Build history of the part. All positions in model axes, mm. Give positions to 0.01 mm unless a question says otherwise; leave off trailing zeros. Loops run counter-clockwise (first coordinate to the right, second up) from the corner with the lowest first, then second, coordinate; pieces in that order, holes last. Notation, with made-up numbers: (-30.75, -21.75) -> (13.25, -21.75) arc R10 cw to (13.25, -12.75) -> close; hole circle Ø5 at (51.25, -10.75). An arc over 180 degrees is marked (long way). Answer in a Markdown table with one row per item. Add a question column.
from build123d import *

# Parameters (mm, degrees)
SKETCH1_W           = 180
SKETCH1_H           = 9.9
BOSS_EXTRUDE1_DEPTH = 4.9
SKETCH2_R           = 1.65
CUT_EXTRUDE1_DEPTH  = 5.9
CUT_EXTRUDE2_DEPTH  = 2.2


with BuildPart() as part:
    # Sketch1 → Boss-Extrude1 (new body)
    with BuildSketch(Plane.XY):
        with Locations((-56.357347179, 33.440788785)):
            Rectangle(SKETCH1_W, SKETCH1_H)
    extrude(amount=-BOSS_EXTRUDE1_DEPTH)

    # Sketch2 → Cut-Extrude1 (cut, through all)
    with BuildSketch(Plane.XY):
        with Locations((-136.357347179, 33.440788785)):
            Circle(SKETCH2_R)
        with Locations((-66.357347179, 33.440788785)):
            Circle(SKETCH2_R)
        with Locations((-46.357347179, 33.440788785)):
            Circle(SKETCH2_R)
        with Locations((23.642652821, 33.440788785)):
            Circle(SKETCH2_R)
    extrude(amount=-CUT_EXTRUDE1_DEPTH, mode=Mode.SUBTRACT)

    # Sketch3 → Cut-Extrude2 (cut)
    with BuildSketch(Plane.XY):
        Polygon((-134.711898912, 30.590788785), (-133.066450645, 33.440788785), (-134.711898912, 36.290788785), (-138.002795446, 36.290788785), (-139.648243713, 33.440788785), (-138.002795446, 30.590788785), align=None)
        Polygon((-64.711898912, 30.590788785), (-63.066450645, 33.440788785), (-64.711898912, 36.290788785), (-68.002795446, 36.290788785), (-69.648243713, 33.440788785), (-68.002795446, 30.590788785), align=None)
        Polygon((-44.711898912, 30.590788785), (-43.066450645, 33.440788785), (-44.711898912, 36.290788785), (-48.002795446, 36.290788785), (-49.648243713, 33.440788785), (-48.002795446, 30.590788785), align=None)
        Polygon((25.288101088, 30.590788785), (26.933549355, 33.440788785), (25.288101088, 36.290788785), (21.997204554, 36.290788785), (20.351756287, 33.440788785), (21.997204554, 30.590788785), align=None)
    extrude(amount=-CUT_EXTRUDE2_DEPTH, mode=Mode.SUBTRACT)


solid = part.part
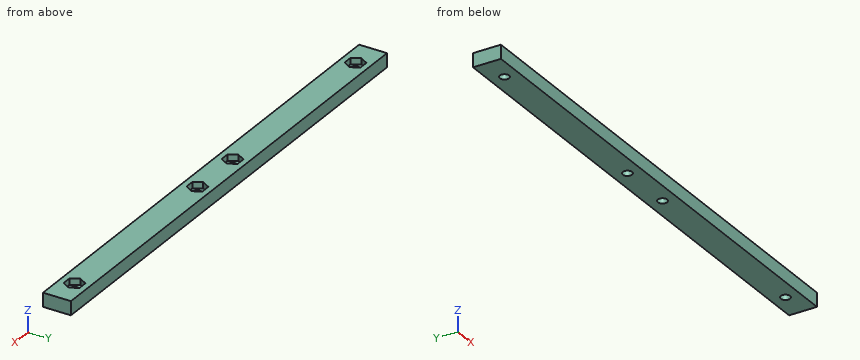
(1) Saw through at A-A, the plane z = -3.15. List the corners of the cut face in (x, y), then the cut area to 3 significant figures.
(2) Flat gauge pin, fed straight in: pin 1 Ø1.7 at (x, y) = (-135, 34) entering from +Z. Where does the tip first touch, or does it go through?
(3) Wall check: line 1 along X through (y, z) = (31.5, -0.6); line 2 along Y through (x, z) = (-136, -0.25); line 3 along X through (y, z) = (36, -0.35). Give the ranges that are in metal, low to high. Write a range as from..to.
Worked answers:
| question | item | result |
|---|---|---|
| 1 | outline | (-146.36, 28.49) -> (33.64, 28.49) -> (33.64, 38.39) -> (-146.36, 38.39) -> close; hole circle Ø3.3 at (-136.36, 33.44); hole circle Ø3.3 at (-66.36, 33.44); hole circle Ø3.3 at (-46.36, 33.44); hole circle Ø3.3 at (23.64, 33.44) |
| 1 | area | 1,750 mm^2 |
| 2 | pin 1 | z = -2.2 |
| 3 | line 1 | -146.36..-138.53, -134.19..-68.53, -64.19..-48.53, -44.19..21.47, 25.81..33.64 |
| 3 | line 2 | 28.49..30.59, 36.29..38.39 |
| 3 | line 3 | -146.36..-138.17, -134.54..-68.17, -64.54..-48.17, -44.54..21.83, 25.46..33.64 |
